The listing builds one solid part. Answer for the finished solid, in the listing's coordinates (mm). A direction names the side the tool comes from. Coordinates: 2 decimals unless noted, no trailing zeros. Loops run counter-clockwise (first coordinate to the right, second up) from the corner with the lowest first, then second, coordinate; pieces in that order, holes last. Notation, with made-up numbers: M 72.5,26 L 83.5,26 A9 cw 83.5,40 Z; hole C 8.25,-30 d1. An arc over 180 degrees is marked long. Answer as a JSON object with one key per item and string values. Group by question number.
1. Given pin 1 (2.5 mm diameter, centred on x = 1, y = 16.5, fed in from -Z), flat-ended and moving along its own axis, determine where the tip first touches the part or whether it passes through.
2. For faces 1 (the face through (-5, 17, 0)), 2 (the face through (-31.33, 13.98, -6.73)), determine the directions among +Z, -Z, +X, -X, +Y, -Y from which every point of the face is accessible in a straight line to the end or side of a thin tool.
3. Determine the mould class of faces 3 (the face through (-29.717, 16, -3)), 4 (the face through (-5, 17, 3.175)), 5 (the face through (21.19, 19.66, -6.73)), 6 (the face through (-31.33, 15.26, -5.39)) for opening direction Z: released by +Z, released by -Z, zero draft, split by the parting line, or undercut.
4. A cutting plane is placed at A-A on z = -1.5. Give the vertices of the cut face in (x, y).
5. A cutting plane is placed at C-C on z = -5.25. Give the vertices of the cut face in (x, y).
6. A cutting plane is placed at B-B on y = 17.75. Give the vertices of the cut face in (x, z) (3 decimals), and give its area (3 significant figures).
7. Straight lines are drawn through the part: L1, parallel to X at y = 17.75, z = -3; L2, parallel to Z at x = -23.5, y = 18.25 (3 decimals). For each, find the intervals that lie inside material, in ascending order.
8. A cutting plane is placed at D-D on y = 14. Give the vertices of the cut face in (x, z) (3 decimals).
from build123d import *

# Parameters (mm, degrees)
F0_W        = 49.2125
F0_H        = 7.9375
F1_DEPTH    = 3.175
F2_DEPTH    = 3.302
F3_DEPTH    = 3.175
F4_W        = 3.175
F4_H        = 7.9375
F5_DEPTH    = 7.9375
F7_D        = 3.2639
F8_T1_DEPTH = 23.114
F8_T3_DEPTH = 23.114


# Not quite as in the source:
# - a fillet or chamfer that OpenCascade refuses, or shapes differently, is made with other operations: its cross-section is extruded or revolved along the edge and cut away or added


with BuildPart() as f1:
    # F0 (on Top) → F1 (new body)
    with BuildSketch(Plane.XY):
        with Locations((-5.1108673215, 16.8213252627)):
            Rectangle(F0_W, F0_H)
    extrude(amount=F1_DEPTH)

    # F2 (add): a face of the model
    f2_faces = [f1.faces().sort_by_distance(p)[0] for p in [
        (19.4953826785, 16.8213252627, 1.5875),
    ]]
    extrude(f2_faces, amount=F2_DEPTH)

    # F3 (add): a face of the model
    f3_faces = [f1.faces().sort_by_distance(p)[0] for p in [
        (-29.7171173215, 16.8213252627, 1.5875),
    ]]
    extrude(f3_faces, amount=F3_DEPTH)

    # F4 (on face) → F5 (join)
    with BuildSketch(Plane(origin=(0, 0, 0), x_dir=(1, 0, 0), z_dir=(0, 0, -1))):
        with Locations((21.2098826785, -16.8213252627)):
            Rectangle(F4_W, F4_H)
        with Locations((-31.3046173215, -16.8213252627)):
            Rectangle(F4_W, F4_H)
    extrude(amount=F5_DEPTH)

    # F7 (through all)
    with Locations(Plane.YZ.offset(22.7973826785)):
        with Locations((16.7667926535, -4.7623126715)):
            Hole(F7_D / 2)

    # F8: fillet of radius 3.9878 on 4 edges, made by hand

    # F8_s2 → F8_t1 (cut)
    with BuildSketch(Plane.YZ.offset(9.6528826785)):
        with BuildLine():
            ThreePointArc((12.8525752627, -3.9497), (14.0205748406, -6.769500422), (16.8403752627, -7.9375))
            Line((16.8403752627, -7.9375), (12.8525752627, -7.9375))
            Line((12.8525752627, -7.9375), (12.8525752627, -3.9497))
        make_face()
        with BuildLine():
            ThreePointArc((20.7900752627, -3.9497), (19.6220756847, -6.769500422), (16.8022752627, -7.9375))
            Line((16.8022752627, -7.9375), (20.7900752627, -7.9375))
            Line((20.7900752627, -7.9375), (20.7900752627, -3.9497))
        make_face()
    extrude(amount=F8_T1_DEPTH, mode=Mode.SUBTRACT)

    # F8_s4 → F8_t3 (cut)
    with BuildSketch(Plane.YZ.offset(-42.8616173215)):
        with BuildLine():
            ThreePointArc((12.8525752627, -3.9497), (14.0205748406, -6.769500422), (16.8403752627, -7.9375))
            Line((16.8403752627, -7.9375), (12.8525752627, -7.9375))
            Line((12.8525752627, -7.9375), (12.8525752627, -3.9497))
        make_face()
        with BuildLine():
            ThreePointArc((20.7900752627, -3.9497), (19.6220756847, -6.769500422), (16.8022752627, -7.9375))
            Line((16.8022752627, -7.9375), (20.7900752627, -7.9375))
            Line((20.7900752627, -7.9375), (20.7900752627, -3.9497))
        make_face()
    extrude(amount=F8_T3_DEPTH, mode=Mode.SUBTRACT)


solid = f1.part
From the geometry:
{
 "1": {"pin 1": "stops at z = 0"},
 "2": {"face 1": "-Z, +Y, -Y", "face 2": "-Z, +X, -X, -Y"},
 "3": {"face 3": "zero draft", "face 4": "released by +Z", "face 5": "released by -Z", "face 6": "undercut"},
 "4": {"outline": "M -32.89,12.85 L -29.72,12.85 L -29.72,20.79 L -32.89,20.79 Z; M 19.62,12.85 L 22.8,12.85 L 22.8,20.79 L 19.62,20.79 Z"},
 "5": {"outline": "M -32.89,13.07 L -29.72,13.07 L -29.72,15.21 L -32.89,15.21 Z; M -32.89,18.32 L -29.72,18.32 L -29.72,20.57 L -32.89,20.57 Z; M 19.62,13.07 L 22.8,13.07 L 22.8,15.21 L 19.62,15.21 Z; M 19.62,18.32 L 22.8,18.32 L 22.8,20.57 L 19.62,20.57 Z"},
 "6": {"outline": "M -32.892,-7.823 L -29.717,-7.823 L -29.717,-6.065 L -32.892,-6.065 Z; M -32.892,-3.46 L -29.717,-3.46 L -29.717,0 L 19.622,0 L 19.622,-3.46 L 22.797,-3.46 L 22.797,3.175 L -32.892,3.175 Z; M 19.622,-7.823 L 22.797,-7.823 L 22.797,-6.065 L 19.622,-6.065 Z", "area": "210 mm²"},
 "7": {"L1": "x = -32.89 to -29.72, 19.62 to 22.8", "L2": "z = 0 to 3.175"},
 "8": {"outline": "M -32.892,-6.749 L -29.717,-6.749 L -29.717,0 L 19.622,0 L 19.622,-6.749 L 22.797,-6.749 L 22.797,3.175 L -32.892,3.175 Z"}
}
